Source: CAD feature listing. Evaluate the final solid. Frame: model axes, mm. A direction names the side the tool comes from. Round coordinates to 2 decimals unless told otherwise and drop trailing zeros. Loops run counter-clockwise (first coordinate to the right, second up) from the corner with the lowest first, then second, coordinate; pieces in that order, holes last. Notation, with made-up numbers: M 79,57 L 130,57 A34 ccw 130,88 Z; hole C -23,44 d10. An arc over 180 degrees is marked long. Answer as a JSON object with one key per item and string values.
from build123d import *

# Parameters (mm, degrees)
SKETCH1_W                                       = 30
SKETCH1_H                                       = 15
CSK_FOR_M3_FLAT_HEAD_MACHINE_SCREW1_D           = 3.6
CSK_FOR_M3_FLAT_HEAD_MACHINE_SCREW1_CSINK_D     = 6.3
CSK_FOR_M3_FLAT_HEAD_MACHINE_SCREW1_CSINK_ANGLE = 90
HOLE1_D                                         = 37
HOLE1_CBORE_D                                   = 46.98238
HOLE1_CBORE_DEPTH                               = 11


with BuildPart() as part:
    # Sketch1 → Revolve1 (revolve)
    with BuildSketch(Plane.XZ, mode=Mode.PRIVATE) as revolve1_sk:
        with Locations((15, 7.5)):
            Rectangle(SKETCH1_W, SKETCH1_H)
    revolve(revolve1_sk.sketch.rotate(Axis((0, 0, 15), (0, 0, -1)), 180), axis=Axis((0, 0, 15), (0, 0, -1)))

    # CSK for M3 Flat Head Machine Screw1 (through all)
    with Locations(Plane(origin=(0, 0, 0), x_dir=(-1, 0, 0), z_dir=(0, 0, -1))):
        with Locations((23.166179551, -13.375), (23.166179551, 13.375), (0, -26.75), (-23.166179551, 13.375), (-23.166179551, -13.375), (0, 26.75)):
            CounterSinkHole(CSK_FOR_M3_FLAT_HEAD_MACHINE_SCREW1_D / 2, CSK_FOR_M3_FLAT_HEAD_MACHINE_SCREW1_CSINK_D / 2, counter_sink_angle=CSK_FOR_M3_FLAT_HEAD_MACHINE_SCREW1_CSINK_ANGLE)

    # Hole1 (through all)
    with Locations(Plane.XY.offset(15)):
        with Locations((0, 0)):
            CounterBoreHole(HOLE1_D / 2, HOLE1_CBORE_D / 2, HOLE1_CBORE_DEPTH)


solid = part.part
Item 1: Line query: probe 1 along Y at (x, z) = (0, 12.25); probe 2 along Y at (x, z) = (0, 2.25); probe 3 along X at (y, z) = (-13.5, 7.5). Output: solid intervals per line, ascending. Write a range as from..to.
Answer sheet:
{"probe 1": "y = -30..-28.55, -24.95..-23.49, 23.49..24.95, 28.55..30", "probe 2": "y = -30..-28.55, -24.95..-18.5, 18.5..24.95, 28.55..30", "probe 3": "x = -26.79..-24.96, -21.37..-19.22, 19.22..21.37, 24.96..26.79"}
Item 2: Pull-direction query (X, two-part tool) for faces 1 (the cylindrical face through (-16.128, 25.296, 7.605)), 2 (the cylindrical face through (10.84, -20.84, 9.58)), 3 (the flat face through (-16, -18, 15)); classes: pulls with the +X half, pulls with the -X half, needs draft (parallel to the pull), parting line crosses it, or undercut.
Answer sheet:
{"face 1": "parting line crosses it", "face 2": "undercut", "face 3": "needs draft"}
Item 3: Access query for faces 4 (the flat face through (-14, -13, 0)), 5 (the flat face through (10, -16, 4)). Directions: +Z, -Z, +X, -X, +Y, -Y. A direction counts if a zero-diameter tool reaches every point of the face in a straight line with its end or side. Return the directions, or none.
Answer sheet:
{"face 4": "-Z, +X, -X, +Y, -Y", "face 5": "+Z"}
Item 4: Contact query for flat-ended pins moving along their axis: pin 1 Ø2 at (x, z) = (-12, 5.5) entering from +Y; pin 2 Ø4 at (x, z) = (-4, 2) entering from +Y; pin 3 Ø4.5 at (x, y) = (0, -26.75) entering from -Z. Output: stop coordinate, or through.
Answer sheet:
{"pin 1": "stops at y = 27.91", "pin 2": "stops at y = 29.93", "pin 3": "stops at z = 0.9"}
Item 5: Section D-D on z = 13. Return the cut outline in (x, y) (3 decimals).
Answer sheet:
{"outline": "C 0,0 d60; hole C -23.166,-13.375 d3.6; hole C -23.166,13.375 d3.6; hole C 0,0 d46.982; hole C 0,-26.75 d3.6; hole C 0,26.75 d3.6; hole C 23.166,-13.375 d3.6; hole C 23.166,13.375 d3.6"}
Item 6: Section A-A on x = 0. Return the cut outline in (y, z).
Answer sheet:
{"outline": "M -30,0 L -29.9,0 L -28.55,1.35 L -28.55,15 L -30,15 Z; M -24.95,1.35 L -23.6,0 L -18.5,0 L -18.5,4 L -23.49,4 L -23.49,15 L -24.95,15 Z; M 18.5,0 L 23.6,0 L 24.95,1.35 L 24.95,15 L 23.49,15 L 23.49,4 L 18.5,4 Z; M 28.55,1.35 L 29.9,0 L 30,0 L 30,15 L 28.55,15 Z"}
Item 7: Section B-B on y = 0. Return the cut outline in (x, z), then the cut area to 3 significant figures.
Answer sheet:
{"outline": "M -30,0 L -18.5,0 L -18.5,4 L -23.49,4 L -23.49,15 L -30,15 Z; M 18.5,0 L 30,0 L 30,15 L 23.49,15 L 23.49,4 L 18.5,4 Z", "area": "235 mm²"}
Item 8: Section C-C on x = -12.5. Return the cut outline in (y, z).
Answer sheet:
{"outline": "M -27.27,0 L -13.64,0 L -13.64,4 L -19.89,4 L -19.89,15 L -27.27,15 Z; M 13.64,0 L 27.27,0 L 27.27,15 L 19.89,15 L 19.89,4 L 13.64,4 Z"}
